Design review of the part built by this model. Coordinates are the model's own, in mm. Face numbers are marked on the shaded views. A direction names the side the tool comes from. Give positions to 0.01 mm unless a question says otherwise; leave off trailing zeros. Loops run counter-clockwise (first coordinate to the right, second up) from the corner with the lowest first, then second, coordinate; pieces in that order, holes last. Notation, with made-up numbers: M 13,89.5 L 18,89.5 A13 ccw 18,93.5 Z; hole C 87.25,0 d6. An arc over 180 degrees is marked long. Use a Markdown table: item, result. Add a question column.
(1) Add section A-A, the plane y = 0. Give the boundary of the cut face in (x, z), then the cut area to 3 significant figures.
(2) For the marked faces 4 and 5, list the 3-axis set-ups (+Z, -Z, +X, -X, +Y, -Y) from which the entire face can be reached by the end or side of a thin tool; tool diameter is ignored.
(3) Add section D-D, the plane y = -8. Give the boundary of the cut face in (x, z), then the cut area to 3 significant figures.
(4) Add section C-C, the plane z = -2.35. Give the boundary of the cut face in (x, y), then the cut area to 3 significant figures.
(5) Draft analysis for pull direction Y (two halves, no side actions). For the marked faces 1, 2 and 3, state which applies: pulls with the +Y half, pulls with the -Y half, needs draft (parallel to the pull), parting line crosses it, or undercut.
(6) For probe 1 along Y at (x, z) = (0, -3.85); probe 2 along Y at (x, z) = (0, 0.9); probe 3 along Z at (x, y) = (9.25, -2), list the stretches that pass through material, from the lowest coordinate up.
(7) Insertion check: pin 1 Ø1.5 at (x, z) = (0, -2) entering from -Y; pin 2 Ø1 at (x, z) = (7.5, -1) entering from +Y; pin 3 Ø2 at (y, z) = (5.5, -3) entering from -X. Each pin has a flat end and moves straight along its axis. Give the tip position at first contact, or say it passes through.
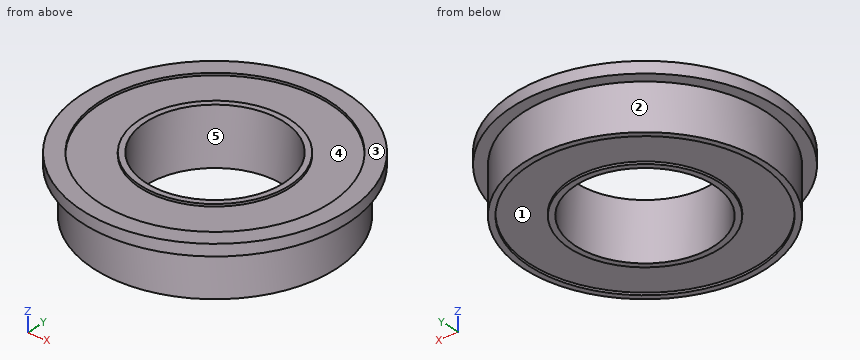
```python
from build123d import *

# Parameters (mm, degrees)
SKETCH_1_R          = 11.5
SKETCH_1_R_2        = 10.5
EXTRUDE_1_DEPTH     = 1
EXTRUDE_START       = -5
SKETCH_2_R          = 10.5
SKETCH_2_R_2        = 6
EXTRUDE_2_DEPTH     = 5
SKETCH_3_R          = 10
SKETCH_3_R_2        = 6.5
CUT_EXTRUDE_1_DEPTH = 0.2


with BuildPart() as part:
    # 草图1 → 凸台-拉伸1 (new body)
    with BuildSketch(Plane.XY):
        Circle(SKETCH_1_R)
        Circle(SKETCH_1_R_2, mode=Mode.SUBTRACT)
    extrude(amount=EXTRUDE_1_DEPTH)

    # 草图2 → 凸台-拉伸2 (add)
    with BuildSketch(Plane.XY.offset(1).offset(EXTRUDE_START)):
        Circle(SKETCH_2_R)
        Circle(SKETCH_2_R_2, mode=Mode.SUBTRACT)
    extrude(amount=EXTRUDE_2_DEPTH)

    # 草图3 → 切除-拉伸1 (cut)
    with BuildSketch(Plane(origin=(0, 0, -4), x_dir=(-1, 0, 0), z_dir=(0, 0, -1))):
        Circle(SKETCH_3_R)
        Circle(SKETCH_3_R_2, mode=Mode.SUBTRACT)
    cut_extrude_1 = extrude(amount=-CUT_EXTRUDE_1_DEPTH, mode=Mode.SUBTRACT)

    # 镜向1: 切除-拉伸1 across plane
    add(cut_extrude_1.mirror(Plane(origin=(0, 0, -1.5), x_dir=(1, 0, 0), z_dir=(0, 0, -1))), mode=Mode.SUBTRACT)


solid = part.part
```
Established:
| question | item | result |
|---|---|---|
| 1 | outline | M -11.5,0 L -10.5,0 L -10.5,-4 L -10,-4 L -10,-3.8 L -6.5,-3.8 L -6.5,-4 L -6,-4 L -6,1 L -6.5,1 L -6.5,0.8 L -10,0.8 L -10,1 L -11.5,1 Z; M 6,-4 L 6.5,-4 L 6.5,-3.8 L 10,-3.8 L 10,-4 L 10.5,-4 L 10.5,0 L 11.5,0 L 11.5,1 L 10,1 L 10,0.8 L 6.5,0.8 L 6.5,1 L 6,1 Z |
| 1 | area | 44.2 mm^2 |
| 2 | face 4 | +Z |
| 2 | face 5 | +Z, -Z |
| 3 | outline | M -8.26,0 L -6.8,0 L -6.8,-4 L -6,-4 L -6,-3.8 L 6,-3.8 L 6,-4 L 6.8,-4 L 6.8,0 L 8.26,0 L 8.26,1 L 6,1 L 6,0.8 L -6,0.8 L -6,1 L -8.26,1 Z |
| 3 | area | 66.1 mm^2 |
| 4 | outline | C 0,0 d21; hole C 0,0 d12 |
| 4 | area | 233 mm^2 |
| 5 | face 1 | undercut |
| 5 | face 2 | parting line crosses it |
| 5 | face 3 | needs draft |
| 6 | probe 1 | -10.5 to -10, -6.5 to -6, 6 to 6.5, 10 to 10.5 |
| 6 | probe 2 | -11.5 to -10, -6.5 to -6, 6 to 6.5, 10 to 11.5 |
| 6 | probe 3 | -3.8 to 0.8 |
| 7 | pin 1 | y = -10.5 |
| 7 | pin 2 | y = 7.83 |
| 7 | pin 3 | x = -9.49 |
